For this review, take the finished solid that the model builds, in its own axes (mm). Face numbers are marked on the shaded views. Give positions to 0.01 mm unless a question says otherwise; leave off trailing zeros. Write each loop counter-clockwise with the first axis right and the second up, starting at its lowest first coordinate (ties: lowest second). Pieces come first, ordered by that corner, then holes. Notation, with made-up numbers: M 47,-11 L 70,-11 A6 cw 70,-7 Z; hole C -32.75,57 d1. An arc over 180 degrees is marked long. Write item = value, one per line.
```python
from build123d import *

# Parameters (mm, degrees)
F0_W = 15
F0_H = 50
F1_W = 4.208725
F1_H = 50.100006


with BuildPart() as f2:
    # F0 (on Front) → F2 (revolve)
    with BuildSketch(Plane.XZ):
        with Locations((-47.5, 0)):
            Rectangle(F0_W, F0_H)
    revolve(axis=Axis((0, 0, 0), (0, 0, -1)))

    # F1 (on Front) → F3 (revolve)
    with BuildSketch(Plane.XZ):
        with Locations((-38.000499, -0.005182)):
            Rectangle(F1_W, F1_H)
    revolve(axis=Axis((0, 0, 0), (0, 0, -1)))


solid = f2.part
```
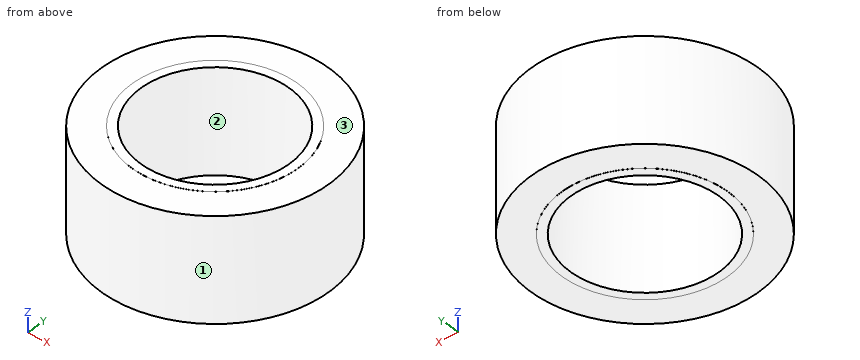
1. The part is to be moulded in two halves that separate along Y. For the marked faces 1, 2 and 3, say which applies: +Y half, -Y half, draft (parallel to the pull), parting line (faces both ways), or undercut.
Responses:
face_1 = parting line
face_2 = undercut
face_3 = draft
2. For line 1 along Z through (x, y) = (32, -33.5); line 2 along Y through (x, z) = (0, 10); line 3 along Y through (x, z) = (-4.5, -5), list the stretches that pass through material, from the lowest coordinate up. Write a range as from..to.
Responses:
line_1 = -25..25
line_2 = -55..-35.9, 35.9..55
line_3 = -54.82..-35.61, 35.61..54.82
3. We need section A-A, the plane x = 0. Write out the cut boundary in (y, z).
Responses:
outline = M -55,-25 L -40.1,-25 L -40.1,-25.06 L -35.9,-25.06 L -35.9,25.04 L -40.1,25.04 L -40.1,25 L -55,25 Z; M 35.9,-25.06 L 40.1,-25.06 L 40.1,-25 L 55,-25 L 55,25 L 40.1,25 L 40.1,25.04 L 35.9,25.04 Z
4. Insertion check: P1, Ø1.5, axis at x = -10.5, z = 19, coming from the -Y side; P2, Ø1.5, axis at x = -32.5, z = 9, coming from the -Y side; P3, Ø8, axis at x = 5.5, y = 30.5, coming from the -Z side; P4, Ø10, axis at x = -17, z = -14.5, coming from the -Y side. Each pin has a flat end and moves straight along its axis. Give the tip position at first contact, or say it passes through.
Responses:
P1 = -54.13
P2 = -44.91
P3 = through
P4 = -53.67
5. We need section C-C, the plane z = 6. Write out the cut boundary in (x, y).
Responses:
outline = C 0,0 d110; hole C 0,0 d71.79
6. We need section D-D, the plane y = 44. Write out the cut boundary in (x, z).
Responses:
outline = M -33,-25 L 33,-25 L 33,25 L -33,25 Z
